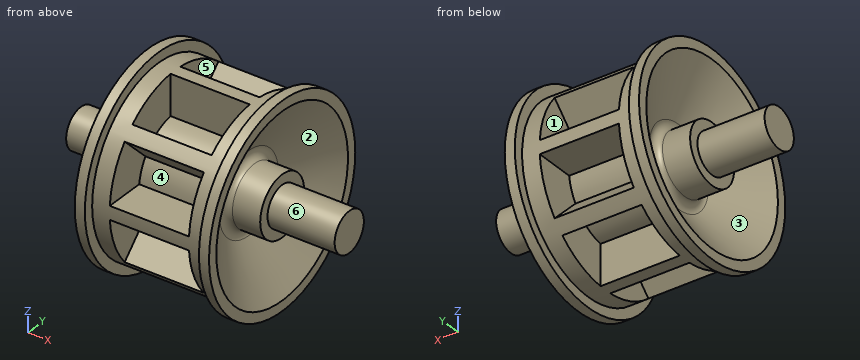
Solid Edge part; units mm, degrees
sketch "Sketch1" plane through (0, 0, 0) normal (0, 0, 1) x (1, 0, 0)
  line L0 (20, -3) -> (10, -3)
  line L1 (10, -3) -> (10, -4.5)
  line L2 (10, -4.5) -> (5.8685, -4.5)
  arc A0 (5.8685, -4.5) -> (5.0365, -6.0547) centre (5.8685, -5.5) ccw
  line L3 (5.0365, -6.0547) -> (10, -13.5)
  line L4 (10, -13.5) -> (10, -15)
  line L5 (8.5, -15) -> (10, -15)
  line L6 (8.5, -13.5) -> (8.5, -15)
  line L7 (0, -13.5) -> (8.5, -13.5)
  line L8 (0, 0) -> (0, -13.5)
  line L9 (0, 0) -> (20, 0)
  line L10 (20, 0) -> (20, -3)
revolve "RevolvedProtrusion1" add sketch "Sketch1" angle 360 about axis through (0, 0, 0) along (1, 0, 0)
sketch "Sketch2" plane through (0, 0, 0) normal (-1, 0, 0) x (0, 0, 1)
  line L0 (-7.433, 1) -> (-19.394, 1)
  line L1 (-19.394, 1) -> (-19.394, 18)
  line L2 (-19.394, 18) -> (-5.9543, 4.5603)
  arc A0 (-5.9543, 4.5603) -> (-7.433, 1) centre (0, 0) ccw
  line L3 (-7.433, -1) -> (-19.394, -1)
  line L4 (-19.394, -1) -> (-19.394, -18)
  line L5 (-19.394, -18) -> (-5.9543, -4.5603)
  arc A1 (-5.9543, -4.5603) -> (-7.433, -1) centre (0, 0) cw
  line L6 (-4.3097, -6.1381) -> (-18, -19.8284)
  line L7 (-18, -19.8284) -> (-1, -19.8284)
  line L8 (-1, -19.8284) -> (-1, -7.433)
  arc A2 (-1, -7.433) -> (-4.3097, -6.1381) centre (0, 0) cw
  line L9 (1, -19.8284) -> (1, -7.433)
  arc A3 (1, -7.433) -> (4.3097, -6.1381) centre (0, 0) ccw
  line L10 (4.3097, -6.1381) -> (18, -19.8284)
  line L11 (18, -19.8284) -> (1, -19.8284)
  line L12 (19.394, -18) -> (5.9543, -4.5603)
  arc A4 (5.9543, -4.5603) -> (7.433, -1) centre (0, 0) ccw
  line L13 (7.433, -1) -> (19.394, -1)
  line L14 (19.394, -1) -> (19.394, -18)
  line L15 (7.433, 1) -> (19.394, 1)
  line L16 (19.394, 1) -> (19.394, 18)
  line L17 (19.394, 18) -> (5.9543, 4.5603)
  arc A5 (5.9543, 4.5603) -> (7.433, 1) centre (0, 0) cw
  line L18 (4.3097, 6.1381) -> (18, 19.8284)
  line L19 (18, 19.8284) -> (1, 19.8284)
  line L20 (1, 19.8284) -> (1, 7.433)
  arc A6 (1, 7.433) -> (4.3097, 6.1381) centre (0, 0) cw
  line L21 (-1, 19.8284) -> (-1, 7.433)
  arc A7 (-1, 7.433) -> (-4.3097, 6.1381) centre (0, 0) ccw
  line L22 (-4.3097, 6.1381) -> (-18, 19.8284)
  line L23 (-18, 19.8284) -> (-1, 19.8284)
extrude "Cutout1" cut sketch "Sketch2" against normal blind 5.9
mirror "Mirror1" about plane through (0, 0, 0) normal (1, 0, 0) of "RevolvedProtrusion1", "Cutout1"
Check sheet for the modelled part. Datum: model origin and axes. Units: mm. Face numbers are marked on the shaded views. A direction names the side the tool comes from. Coordinates: 2 decimals unless noted, no trailing zeros. Order: outer loops, then holes, each group sorted by start corner. A loop starts at its lowest first (then second) coordinate and runs counter-clockwise, first axis right, second up. Notation, with made-up numbers: (-15, -25) -> (18, -25) arc R23 cw to (18, 12) -> close; hole circle Ø11 at (2, -32). An arc over 180 degrees is marked (long way). Write item = value, one per line. Start each with the question number.
1) Cross-section at C-C (x = -16.5). Enter the section's corners in (y, z), then the cut area to 3 significant figures.
2) Material ranges on L1, parallel to X at y = 2.75, z = 13.75; L2, parallel to Z at x = -5.5, y = 3; L3, parallel to Z at x = 7, y = 3.5, recorded low to high.
3) Cross-section at B-B (y = -9.5). State how many separate pieces and enclosed holes the cut face has, then the cut area to 3 significant figures.
4) Go/stop test with flat-tipped pins: P1, Ø5, axis at x = -1, y = -12, coming from the -Z side; P2, Ø3.5, axis at y = 8, z = -4, coming from the +X side; P3, Ø2, axis at y = -9, z = -4, coming from the +X side. Record where each tip stops, or that it passes through.
5) Mould release check, pull along X, two halves, no side actions. Record for the marked faces 1, 2 and 3: +X half, -X half, draft (parallel to the pull), parting line (faces both ways), or undercut.
6) Access from +Z, -Z, +X, -X, +Y, -Y to the whole of each face (thin tool, end or side, straight path). Record for the marked faces 4, 5 and 6.
Ans:
q1.outline = circle Ø6 at (0, 0)
q1.area = 28.3 mm²
q2.L1 = -10 to -8.5, 8.5 to 10
q2.L2 = -6.87 to -6.05, -3.45 to 3.45, 6.05 to 6.87
q2.L3 = -13.04 to -8.29, -2.83 to 2.83, 8.29 to 13.04
q3.separate_pieces = 1
q3.enclosed_holes = 2
q3.area = 173 mm²
q4.P1 = -9.59
q4.P2 = 8.13
q4.P3 = 8.23
q5.face_1 = undercut
q5.face_2 = +X half
q5.face_3 = -X half
q6.face_4 = -Y
q6.face_5 = +Z
q6.face_6 = +X
